Part model, mm, in its own coordinate system. Face numbers are marked on the shaded views. A direction names the side the tool comes from. Coordinates: 2 decimals unless noted, no trailing zeros. Order: outer loops, then holes, each group sorted by start corner. A loop starts at its lowest first (then second) coordinate and runs counter-clockwise, first axis right, second up. Notation, with made-up numbers: M -24.75,-37.75 L 20.25,-37.75 A26 cw 20.25,-8.75 Z; hole C -39.5,-40 d2. An arc over 180 degrees is marked long. Answer in a Markdown table with one row per item. Add a question column.
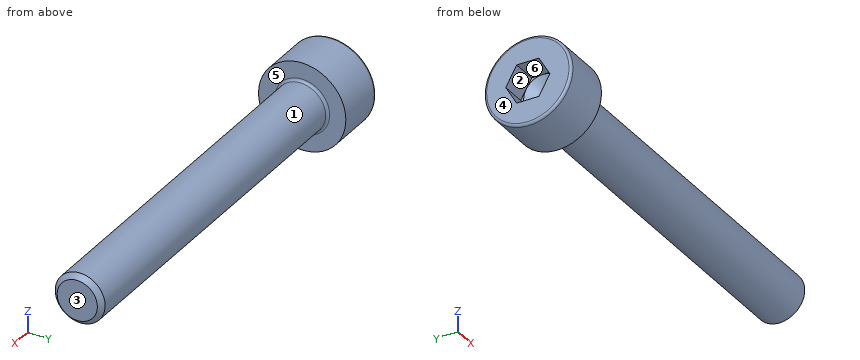
from build123d import *

# Parameters (mm, degrees)
FILLET1_R   = 0.2
FILLET2_R   = 0.2
HEX_2_DEPTH = 2


with BuildPart() as part:
    # BodySke → Base-Revolve (revolve)
    with BuildSketch(Plane.XY, mode=Mode.PRIVATE) as base_revolve_sk:
        Polygon((0, 0), (0, 3.5), (4, 3.5), (4, 2), (33.61, 2), (34, 1.61), (34, 0), align=None)
    revolve(base_revolve_sk.sketch.rotate(Axis((-31.75, 0, 0), (1, 0, 0)), 90), axis=Axis((-31.75, 0, 0), (1, 0, 0)))  # turned: the seam where the file's is

    # Fillet1
    fillet1_edges = [part.edges().sort_by_distance(p)[0] for p in [
        (4, 0, -2),
    ]]
    fillet(fillet1_edges, radius=FILLET1_R)

    # Fillet2
    fillet2_edges = [part.edges().sort_by_distance(p)[0] for p in [
        (0, 0, -3.5),
    ]]
    fillet(fillet2_edges, radius=FILLET2_R)

    # Sketch2 → Hex-PreBroach (revolve, cut)
    with BuildSketch(Plane.XY, mode=Mode.PRIVATE) as hex_prebroach_sk:
        Polygon((0, 1.5355), (2, 1.5355), (2.886521338, 0), (0, 0), align=None)
    revolve(hex_prebroach_sk.sketch.rotate(Axis((0, 0, 0), (1, 0, 0)), 90), axis=Axis((0, 0, 0), (1, 0, 0)), mode=Mode.SUBTRACT)  # turned: the seam where the file's is

    # Sketch3 → Hex 2 (cut)
    with BuildSketch(Plane(origin=(0, 0, 0), x_dir=(0, 0.5, 0.866025404), z_dir=(-1, 0, 0))):
        Polygon((0.886521338, 1.5355), (-0.886521338, 1.5355), (-1.773042677, 0), (-0.886521338, -1.5355), (0.886521338, -1.5355), (1.773042677, 0), align=None)
    extrude(amount=-HEX_2_DEPTH, mode=Mode.SUBTRACT)


solid = part.part
(1) Slice it at A-A (x = 6). List the corners of the cut face in (y, z).
(2) 3-axis set-ups, long thin cutter, end or side, ignore diameter. For the marked faces 4, 5 and 6: which of +Z, -Z, +X, -X, +Y, -Y reach the whole face in a straight line?
(3) Pull direction Y, two halves, no side cores. Call the marked faces 1, 2 and 3: pulls with the +Y half, pulls with the -Y half, needs draft (parallel to the pull), parting line crosses it, or undercut.
(4) Drop flat-ended pins along their axis: P1, Ø1, axis at x = 5.5, z = -1.5, coming from the +Y side; P2, Ø1.5, axis at x = 4.5, z = -2.5, coming from the +Y side; P3, Ø4, axis at x = 28.5, z = 1.5, coming from the -Y side. Give the stop position or say it passes through.
(5) Wall check: line 1 (X direction, y = 2.25, z = 2); line 2 (Y direction, x = 26.5, z = 0); line 3 (Z direction, x = 7.5, y = 1.5). Give the ranges that are in metal, low to high.
Computed:
| question | item | result |
|---|---|---|
| 1 | outline | C 0,0 d4 |
| 2 | face 4 | +Z, -Z, -X, +Y, -Y |
| 2 | face 5 | +X |
| 2 | face 6 | -X |
| 3 | face 1 | parting line crosses it |
| 3 | face 2 | undercut |
| 3 | face 3 | needs draft |
| 4 | P1 | stops at y = 1.73 |
| 4 | P2 | stops at y = 2.91 |
| 4 | P3 | stops at y = -2 |
| 5 | line 1 | x = 0 to 4 |
| 5 | line 2 | y = -2 to 2 |
| 5 | line 3 | z = -1.32 to 1.32 |
